Model file for the job. Use its own axes, mm. A direction names the side the tool comes from. Round coordinates to 2 decimals unless told otherwise and drop trailing zeros. Order: outer loops, then holes, each group sorted by start corner. A loop starts at its lowest first (then second) coordinate and runs counter-clockwise, first axis right, second up. Notation, with made-up numbers: (46.5, 84.5) - (51.5, 84.5) arc R20 cw to (51.5, 96.5) - close; hole circle Ø7 at (-26.5, 55.5). An arc over 180 degrees is marked (long way). Put each result on its own line as item: value. Start each with the question number.
Item 1: Pin check, flat tips, straight feed: pin 1 Ø5 at (y, z) = (-15.5, 4) entering from +X; pin 2 Ø1.5 at (x, y) = (-14.5, -19) entering from -Z; pin 3 Ø5 at (x, z) = (-19.5, 2.5) entering from +Y; pin 4 Ø12 at (x, y) = (0, 0) entering from +Z. Stop position of each tip, or through.
Item 2: Saw through at D-D on x = -21. List the corners of the cut face in (y, z), plus the area to 3 significant figures.
Item 3: Saw through at A-A on x = 19.5. List the corners of the cut face in (y, z), plus the area to 3 significant figures.
Item 4: Saw through at C-C on z = 8.25. List the corners of the cut face in (x, y).
Item 5: Mould opens along X. For faces 1 (the face through (0, 14, 5)), 2 (the face through (0, 0, 3)), 3 (the face through (14, -13, 5)) say: pulls with the +X half, pulls with the -X half, needs draft (parallel to the pull), parting line crosses it, or undercut.
Item 6: Which spindle directions (+Z, -Z, +X, -X, +Y, -Y) get a long thin tool onto all of the face, cutting with end or side? Do faces 4 (the face through (17, -26.952, 4)), 5 (the face through (-7.493, 0.33, 6.549)), 6 (the face through (-17, -26.952, 4)). Say none if no direction does.
Item 7: Probe probe 1 along X at (y, z) = (-28.25, 5); probe 2 along Y at (x, z) = (0, 7.25); probe 3 along Z at (x, y) = (19.5, -28.2). List the from-to ranges inside material, lowest first.
Item 8: Saw through at B-B on z = 5. List the corners of the cut face in (x, y), plus the area to 3 significant figures.
Autodesk Inventor part; units mm, degrees
ref_plane "YZ Plane" through (0, 0, 0) normal (1, 0, 0) x (0, 1, 0)
ref_plane "XZ Plane" through (0, 0, 0) normal (0, 1, 0) x (-1, 0, 0)
ref_plane "XY Plane" through (0, 0, 0) normal (0, 0, 1) x (1, 0, 0)
sketch "Boceto1" plane through (0, 0, 0) normal (0, 0, 1) x (1, 0, 0)
  arc A0 (0, 14) -> (-14, 0) centre (0, 0) ccw
  line L0 (-14, 0) -> (-14, -26.9516)
  line L1 (-14, -26.9516) -> (-25, -26.9516)
  line L2 (-25, -26.9516) -> (-25, -30.9943)
  line L3 (-25, -30.9943) -> (0, -30.9943)
  line L4 (0, -30.9943) -> (0, 14) construction
  arc A1 (0, 7.5) -> (0, -7.5) centre (0, 0) ccw
  arc A2 (14, 0) -> (0, 14) centre (0, 0) ccw
  line L5 (14, 0) -> (14, -26.9516)
  line L6 (14, -26.9516) -> (25, -26.9516)
  line L7 (25, -26.9516) -> (25, -30.9943)
  line L8 (25, -30.9943) -> (0, -30.9943)
  arc A3 (0, -7.5) -> (0, 7.5) centre (0, 0) ccw
  dimension "d2" = 7.5
  dimension "d6" = 50
  dimension "d7" = 28
extrude "Extrusión1" add sketch "Boceto1" along normal blind 10 contours A2 L5 L6 L7 L8 L3 L2 L1 L0 A0 | A3 A1
sketch "Boceto2" plane through (-25, -26.9516, 0) normal (0, 1, 0) x (1, 0, 0)
  line L0 (11, 0) -> (39, 0)
  line L1 (0, -10) -> (50, -10)
  line L2 (11, 0) -> (0, -10)
  line L3 (11, -10) -> (39, -10)
  line L4 (0, 0) -> (50, 0)
  line L5 (11, -10) -> (0, 0)
  line L6 (0, 0) -> (50, -10)
  line L7 (0, -10) -> (50, 0)
  line L8 (25, -5) -> (25, 11.6359)
  circle A0 centre (5.5, -5) radius 2.5
  circle A1 centre (44.5, -5) radius 2.5
  point P0 (25, 0)
  dimension "d3" = 5
extrude "Extrusión2" cut sketch "Boceto2" against normal blind 5 contours A0 L5 L2 | L2 L5 A0 | L5 L2 A0 | L5 A0 L2 | A1
sketch "Boceto3" plane through (0, 0, 10) normal (0, 0, 1) x (1, 0, 0)
  circle A0 centre (0, 0) radius 7.5
  dimension "d8" = 15
extrude "Extrusión3" cut sketch "Boceto3" against normal blind 7
properties part number "sopoetellantas"
Results found:
1. pin 1: stops at x = 14
1. pin 2: stops at z = 0
1. pin 3: stops at y = -26.95
1. pin 4: stops at z = 3
2. outline: (-30.99, 0) - (-26.95, 0) - (-26.95, 3) - (-30.99, 3) - close; (-30.99, 7) - (-26.95, 7) - (-26.95, 10) - (-30.99, 10) - close
2. area: 24.3 mm²
3. outline: (-30.99, 0) - (-26.95, 0) - (-26.95, 2.5) - (-30.99, 2.5) - close; (-30.99, 7.5) - (-26.95, 7.5) - (-26.95, 10) - (-30.99, 10) - close
3. area: 20.2 mm²
4. outline: (-25, -30.99) - (25, -30.99) - (25, -26.95) - (14, -26.95) - (14, 0) arc R14 ccw to (-14, 0) - (-14, -26.95) - (-25, -26.95) - close; hole circle Ø15 at (0, 0)
5. face 1: parting line crosses it
5. face 2: undercut
5. face 3: pulls with the +X half
6. face 4: +Z, -Z, +X, +Y
6. face 5: +Z
6. face 6: +Z, -Z, -X, +Y
7. probe 1: x = -25 to -22, -17 to 17, 22 to 25
7. probe 2: y = -30.99 to -7.5, 7.5 to 14
7. probe 3: z = 0 to 2.5, 7.5 to 10
8. outline: (-25, -30.99) - (-22, -30.99) - (-22, -26.95) - (-25, -26.95) - close; (-17, -30.99) - (17, -30.99) - (17, -26.95) - (14, -26.95) - (14, 0) arc R14 ccw to (-14, 0) - (-14, -26.95) - (-17, -26.95) - close; (22, -30.99) - (25, -30.99) - (25, -26.95) - (22, -26.95) - close; hole circle Ø15 at (0, 0)
8. area: 1,050 mm²
